Design review of the part built by this model. Coordinates are the model's own, in mm. Face numbers are marked on the shaded views. A direction names the side the tool comes from. Give positions to 0.01 mm unless a question says otherwise; leave off trailing zeros. Order: outer loops, then holes, each group sorted by start corner. A loop starts at its lowest first (then second) coordinate and runs counter-clockwise, first axis right, second up. Notation, with made-up numbers: M -11,2.5 L 24,2.5 A27 cw 24,39.5 Z; hole C -28.75,8 d8. An arc over 180 degrees is marked long. Put each result on its own line as item: value. Start each with the question number.
Autodesk Inventor part; units mm, degrees
ref_plane "YZ Plane" through (0, 0, 0) normal (1, 0, 0) x (0, 1, 0)
ref_plane "XZ Plane" through (0, 0, 0) normal (0, 1, 0) x (-1, 0, 0)
ref_plane "XY Plane" through (0, 0, 0) normal (0, 0, 1) x (1, 0, 0)
sketch "Esboço1" plane through (0, 0, 0) normal (0, 1, 0) x (-1, 0, 0)
  line L0 (215, 90) -> (-215, 90)
  line L1 (-215, 90) -> (-215, -90)
  line L2 (-215, -90) -> (215, -90)
  line L3 (215, -90) -> (215, 90)
  point P0 (0, 0)
  dimension "d3" = 180
  dimension "d5" = 215
  dimension "d6" = 430
  dimension "d7" = 90
extrude "Extrusão1" add sketch "Esboço1" along normal blind 2
sketch "Esboço2" plane through (0, 0, 0) normal (0, -1, 0) x (1, 0, 0)
  line L0 (215, -90) -> (-215, -90)
  line L1 (-215, -90) -> (-215, -89.25)
  line L2 (-215, -90) -> (-215, 90)
  line L3 (-215, -89.25) -> (215, -89.25)
  line L4 (215, 90) -> (215, -90)
  line L5 (215, -89.25) -> (215, -90)
  line L6 (215, -90) -> (-215, -90)
  point P0 (0, 0)
  dimension "d10" = 0.75
  dimension "d11" = 430
extrude "Extrusão2" add sketch "Esboço2" along normal blind 2
sketch "Esboço3" plane through (0, 2, 0) normal (0, 1, 0) x (1, 0, 0)
  line L0 (-215, 90) -> (215, 90)
  line L1 (-215, 80) -> (215, 80) construction
  line L2 (-215, 80) -> (-215, 60) construction
  line L3 (-215, 60) -> (215, 60) construction
  line L4 (215, 80) -> (215, 60) construction
  line L5 (-185, 60) -> (-182, 60) construction
  line L6 (-182, 60) -> (-182, 80) construction
  line L7 (-182, 80) -> (-185, 80) construction
  line L8 (-185, 80) -> (-185, 60) construction
  line L9 (-183.5, 60) -> (-183.5, 80) construction
  line L10 (-182, 61.5) -> (-182, 78.5)
  line L11 (-185, 78.5) -> (-185, 61.5)
  arc A0 (-185, 61.5) -> (-182, 61.5) centre (-183.5, 61.5) ccw
  arc A1 (-182, 78.5) -> (-185, 78.5) centre (-183.5, 78.5) ccw
  line L12 (-179, 78.5) -> (-179, 61.5)
  arc A2 (-176, 78.5) -> (-179, 78.5) centre (-177.5, 78.5) ccw
  line L13 (-176, 61.5) -> (-176, 78.5)
  arc A3 (-179, 61.5) -> (-176, 61.5) centre (-177.5, 61.5) ccw
  line L14 (-173, 78.5) -> (-173, 61.5)
  arc A4 (-170, 78.5) -> (-173, 78.5) centre (-171.5, 78.5) ccw
  line L15 (-170, 61.5) -> (-170, 78.5)
  arc A5 (-173, 61.5) -> (-170, 61.5) centre (-171.5, 61.5) ccw
  line L16 (-167, 78.5) -> (-167, 61.5)
  arc A6 (-164, 78.5) -> (-167, 78.5) centre (-165.5, 78.5) ccw
  line L17 (-164, 61.5) -> (-164, 78.5)
  arc A7 (-167, 61.5) -> (-164, 61.5) centre (-165.5, 61.5) ccw
  line L18 (-161, 78.5) -> (-161, 61.5)
  arc A8 (-158, 78.5) -> (-161, 78.5) centre (-159.5, 78.5) ccw
  line L19 (-158, 61.5) -> (-158, 78.5)
  arc A9 (-161, 61.5) -> (-158, 61.5) centre (-159.5, 61.5) ccw
  line L20 (-155, 78.5) -> (-155, 61.5)
  arc A10 (-152, 78.5) -> (-155, 78.5) centre (-153.5, 78.5) ccw
  line L21 (-152, 61.5) -> (-152, 78.5)
  arc A11 (-155, 61.5) -> (-152, 61.5) centre (-153.5, 61.5) ccw
  line L22 (-149, 78.5) -> (-149, 61.5)
  arc A12 (-146, 78.5) -> (-149, 78.5) centre (-147.5, 78.5) ccw
  line L23 (-146, 61.5) -> (-146, 78.5)
  arc A13 (-149, 61.5) -> (-146, 61.5) centre (-147.5, 61.5) ccw
  line L24 (-143, 78.5) -> (-143, 61.5)
  arc A14 (-140, 78.5) -> (-143, 78.5) centre (-141.5, 78.5) ccw
  line L25 (-140, 61.5) -> (-140, 78.5)
  arc A15 (-143, 61.5) -> (-140, 61.5) centre (-141.5, 61.5) ccw
  line L26 (-137, 78.5) -> (-137, 61.5)
  arc A16 (-134, 78.5) -> (-137, 78.5) centre (-135.5, 78.5) ccw
  line L27 (-134, 61.5) -> (-134, 78.5)
  arc A17 (-137, 61.5) -> (-134, 61.5) centre (-135.5, 61.5) ccw
  line L28 (185, 60) -> (182, 60) construction
  line L29 (182, 60) -> (182, 80) construction
  line L30 (182, 80) -> (185, 80) construction
  line L31 (185, 80) -> (185, 60) construction
  line L32 (183.5, 80) -> (183.5, 60) construction
  line L33 (182, 78.5) -> (182, 61.5)
  line L34 (185, 61.5) -> (185, 78.5)
  arc A18 (185, 78.5) -> (182, 78.5) centre (183.5, 78.5) ccw
  arc A19 (182, 61.5) -> (185, 61.5) centre (183.5, 61.5) ccw
  arc A20 (179, 78.5) -> (176, 78.5) centre (177.5, 78.5) ccw
  line L35 (179, 61.5) -> (179, 78.5)
  line L36 (176, 78.5) -> (176, 61.5)
  arc A21 (176, 61.5) -> (179, 61.5) centre (177.5, 61.5) ccw
  arc A22 (173, 78.5) -> (170, 78.5) centre (171.5, 78.5) ccw
  line L37 (173, 61.5) -> (173, 78.5)
  line L38 (170, 78.5) -> (170, 61.5)
  arc A23 (170, 61.5) -> (173, 61.5) centre (171.5, 61.5) ccw
  arc A24 (167, 78.5) -> (164, 78.5) centre (165.5, 78.5) ccw
  line L39 (167, 61.5) -> (167, 78.5)
  line L40 (164, 78.5) -> (164, 61.5)
  arc A25 (164, 61.5) -> (167, 61.5) centre (165.5, 61.5) ccw
  arc A26 (161, 78.5) -> (158, 78.5) centre (159.5, 78.5) ccw
  line L41 (161, 61.5) -> (161, 78.5)
  line L42 (158, 78.5) -> (158, 61.5)
  arc A27 (158, 61.5) -> (161, 61.5) centre (159.5, 61.5) ccw
  arc A28 (155, 78.5) -> (152, 78.5) centre (153.5, 78.5) ccw
  line L43 (155, 61.5) -> (155, 78.5)
  line L44 (152, 78.5) -> (152, 61.5)
  arc A29 (152, 61.5) -> (155, 61.5) centre (153.5, 61.5) ccw
  arc A30 (149, 78.5) -> (146, 78.5) centre (147.5, 78.5) ccw
  line L45 (149, 61.5) -> (149, 78.5)
  line L46 (146, 78.5) -> (146, 61.5)
  arc A31 (146, 61.5) -> (149, 61.5) centre (147.5, 61.5) ccw
  arc A32 (143, 78.5) -> (140, 78.5) centre (141.5, 78.5) ccw
  line L47 (143, 61.5) -> (143, 78.5)
  line L48 (140, 78.5) -> (140, 61.5)
  arc A33 (140, 61.5) -> (143, 61.5) centre (141.5, 61.5) ccw
  arc A34 (137, 78.5) -> (134, 78.5) centre (135.5, 78.5) ccw
  line L49 (137, 61.5) -> (137, 78.5)
  line L50 (134, 78.5) -> (134, 61.5)
  arc A35 (134, 61.5) -> (137, 61.5) centre (135.5, 61.5) ccw
  point P0 (0, 0)
  point P1 (-183.5, 70)
  point P2 (183.5, 70)
  dimension "d15" = 430
  dimension "d16" = 20
  dimension "d19" = 6
  dimension "d26" = 6
  dimension "d31" = 20
  dimension "d33" = 3
  dimension "d35" = 15
  dimension "d37" = 1.5
  dimension "d38" = 20
  dimension "d39" = 3
  dimension "d40" = 30
  dimension "d41" = 30
  dimension "d42" = 10
  dimension "d43" = 1.5
extrude "Extrusão3" cut sketch "Esboço3" against normal blind 4
sketch "Esboço4" plane through (215, 2, 90) normal (1, 0, 0) x (0, 0, -1)
  line L0 (179.25, -4) -> (180, -4)
  line L1 (180, -4) -> (181.2, -4)
  line L2 (181.2, -4) -> (181.2, 0)
  line L3 (181.2, 0) -> (180, 0)
  line L4 (0, 0) -> (180, 0)
  line L5 (180, 0) -> (180, -4)
  point P0 (90, -2)
  dimension "d46" = 1.2
  dimension "d47" = 4
extrude "Extrusão4" add sketch "Esboço4" against normal blind 430
equation "\"d3\" = 2 * d7"
equation "\"d6\" = 2 * d5"
properties material "Aço, carbono"
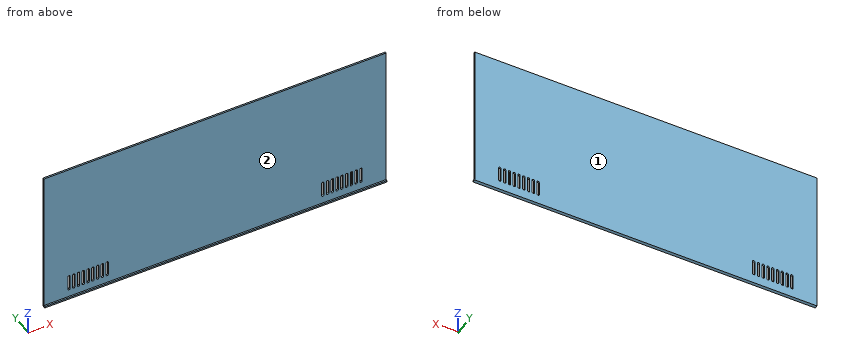
1. Consider section C-C on y = -0.65. Give the boundary of the cut face in (x, z), then the cut area to 4 significant figures.
2. Insertion check: pin 1 (1 mm diameter, centred on x = -129, z = -12.5, fed in from -Y). The pin has a flat end and moves straight along its axis. Give the tip position at first contact, or say it passes through.
3. Consider section B-B on z = -30.5. Give the boundary of the cut face in (x, y), then the cut area to 3 significant figures.
4. Machinability: for the marked faces 1 and 2, which of the approach directions +Z, -Z, +X, -X, +Y, -Y give a long, thin tool a straight path to every point of the face, cutting with its end or side? Answer none if there is none.
5. Consider section A-A on x = 13. Give the boundary of the cut face in (y, z), then the cut area to 3 significant figures.
6. To check wall thickness, follow probe 1 along Z at (x, y) = (167, -1.15); probe 2 along Y at (x, z) = (-27, 51). State the ranges of each line that lie inside material, in increasing order.
Returned:
1. outline: M -215,-91.2 L 215,-91.2 L 215,-89.25 L -215,-89.25 Z
1. area: 838.5 mm2
2. pin 1: stops at y = 0
3. outline: M -215,0 L 215,0 L 215,2 L -215,2 Z
3. area: 860 mm2
4. face 1: +Z, -Z, +X, -X, +Y
4. face 2: +Z, +X, -X, -Y
5. outline: M -2,-91.2 L 2,-91.2 L 2,90 L 0,90 L 0,-89.25 L -2,-89.25 Z
5. area: 366 mm2
6. probe 1: z = -91.2 to -89.25
6. probe 2: y = 0 to 2
